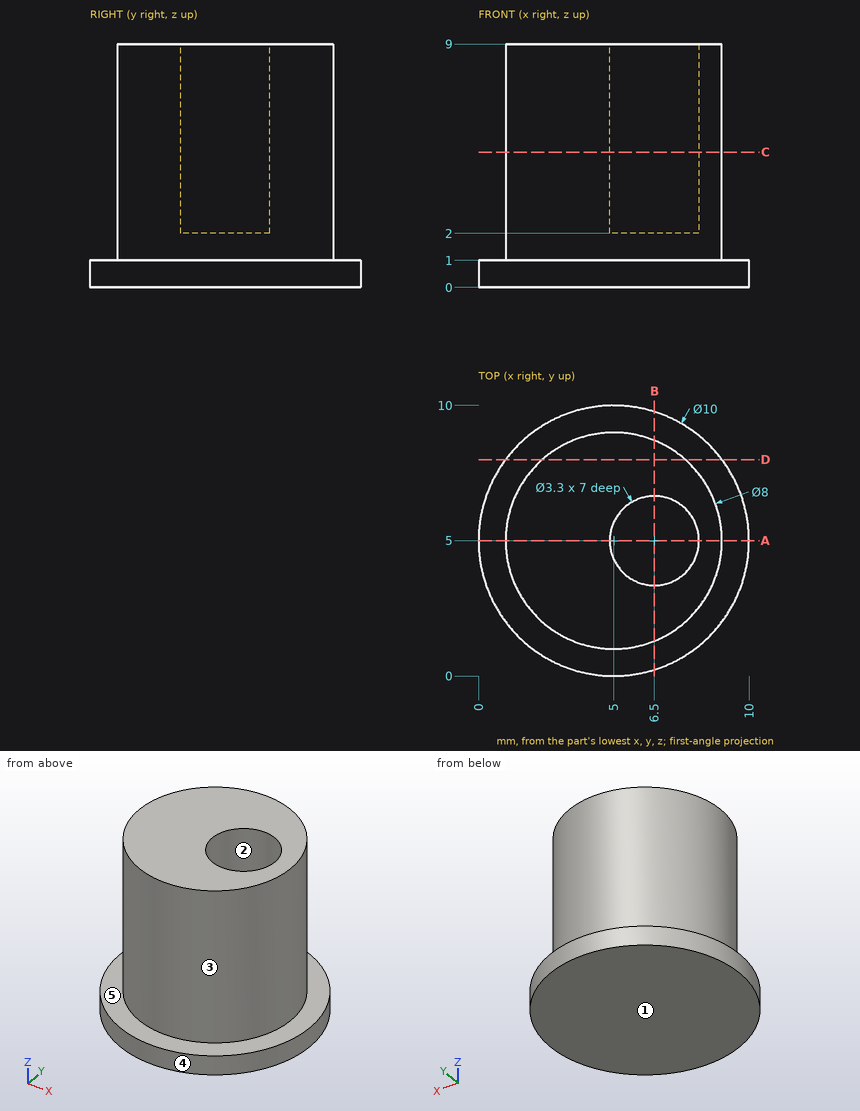
Study the drawing (mm; zero at the part's minimum x, y, z) and answer. A direction names the side the tool comes from. Give positions to 0.01 mm unless a question says otherwise; leave off trailing zeros. Loops run counter-clockwise (first coordinate to the right, second up) from the corner with the lowest first, then second, coordinate; pieces in that order, holes last. Notation, with made-up numbers: (43, -28) - (65, -28) arc R11 ccw to (65, -13) - close; hole circle Ø11 at (75, 28.5). An arc over 180 degrees is marked (long way). Answer as CSV lines item,"result". Start each with the question number.
1) Determine the mould class of the marked faces 1, 2 and 3 for opening direction X: released by +X, released by -X, zero draft, split by the parting line, or undercut.
2) Find section D-D (y = 8). Write down the section's boundary in (x, z), then the cut area to 3 significant figures.
3) Find section B-B (x = 6.5). Write down the section's boundary in (y, z), then the cut area to 3 significant figures.
4) Each of these flat-tipped pins is pushed along its axis until it touches: pin 1 Ø1 at (y, z) = (7.5, 3.5) entering from -X; pin 2 Ø5 at (x, z) = (2.5, 2) entering from -Y; pin 3 Ø2 at (x, z) = (2, 3.5) entering from -Y. Where does it stop, or does it pass through?
5) Find section A-A (y = 5). Write down the section's boundary in (x, z), then the cut area to 3 significant figures.
6) Find section C-C (z = 5). Write down the section's boundary in (x, y), then the cut area to 3 significant figures.
7) Which of the six approach directions +Z, -Z, +X, -X, +Y, -Y give full straight-line access (tool end or side, diameter ignored) to the marked faces 4 and 5?
8) Straight lines are drawn through the part: L1, parallel to Z at x = 7.25, y = 1; L2, parallel to Z at x = 6, y = 5.5; L3, parallel to X at y = 5.5, z = 4.5. For each, find the intervals that lie inside material, in ascending order. Write a range as from..to.
Findings below:
1,face 1,"zero draft"
1,face 2,"undercut"
1,face 3,"split by the parting line"
2,outline,"(1, 0) - (9, 0) - (9, 1) - (7.65, 1) - (7.65, 9) - (2.35, 9) - (2.35, 1) - (1, 1) - close"
2,area,"50.3 mm^2"
3,outline,"(0.23, 0) - (9.77, 0) - (9.77, 1) - (8.71, 1) - (8.71, 9) - (6.65, 9) - (6.65, 2) - (3.35, 2) - (3.35, 9) - (1.29, 9) - (1.29, 1) - (0.23, 1) - close"
3,area,"45.8 mm^2"
4,pin 1,"x = 1.54"
4,pin 2,"y = 0"
4,pin 3,"y = 1.54"
5,outline,"(0, 0) - (10, 0) - (10, 1) - (9, 1) - (9, 9) - (8.15, 9) - (8.15, 2) - (4.85, 2) - (4.85, 9) - (1, 9) - (1, 1) - (0, 1) - close"
5,area,"50.9 mm^2"
6,outline,"circle Ø8 at (5, 5); hole circle Ø3.3 at (6.5, 5)"
6,area,"41.7 mm^2"
7,face 4,"+Z, -Z"
7,face 5,"+Z"
8,L1,"0..1"
8,L2,"0..2"
8,L3,"1.03..4.93, 8.07..8.97"
